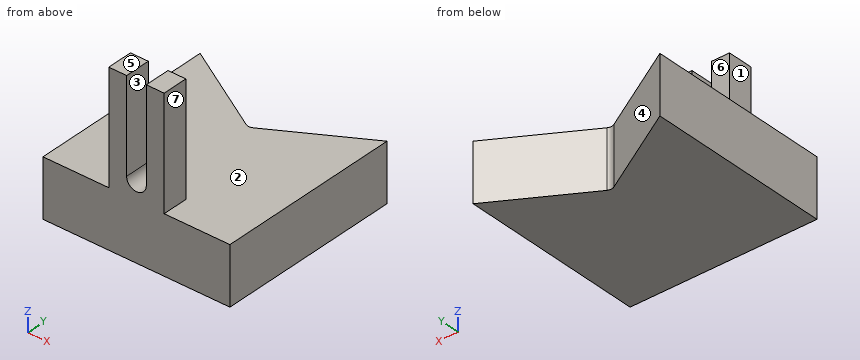
```python
from build123d import *

# Parameters (mm, degrees)
BOSS_EXTRUDE1_DEPTH      = 20.7518
BOSS_EXTRUDE3_DEPTH      = 10
BOSS_EXTRUDE3_DEPTH_BACK = 10
SKETCH6_W                = 40
SKETCH6_H                = 9.27
FILLET1_R                = 2.54
CUT_EXTRUDE11_START      = -47.652475
CUT_EXTRUDE11_DEPTH      = 10


with BuildPart() as part:
    # Sketch1 → Boss-Extrude1 (new body)
    with BuildSketch(Plane.XY):
        Polygon((-33.735, 19.476911331), (0, 0), (33.735, 19.476911331), (33.735, -47.652474646), (-33.735, -47.652474646), align=None)
    extrude(amount=BOSS_EXTRUDE1_DEPTH)

    # Sketch6 → Boss-Extrude3 (add, two sides: drawn at the far end of the back side and taken through both)
    with BuildSketch(Plane(origin=(0, 0, 0), x_dir=(0, 0, -1), z_dir=(1, 0, 0)).offset(-BOSS_EXTRUDE3_DEPTH_BACK)):
        with Locations((-40.7518, -43.017474646)):
            Rectangle(SKETCH6_W, SKETCH6_H)
    extrude(amount=BOSS_EXTRUDE3_DEPTH + BOSS_EXTRUDE3_DEPTH_BACK)

    # Fillet1
    fillet1_edges = [part.edges().sort_by_distance(p)[0] for p in [
        (0, 0, 10.3759),
    ]]
    fillet(fillet1_edges, radius=FILLET1_R)

    # Sketch7 → Cut-Extrude11 (cut)
    with BuildSketch(Plane(origin=(0, 0, 0), x_dir=(1, 0, 0), z_dir=(0, 1, 0)).offset(CUT_EXTRUDE11_START)):
        with BuildLine():
            Line((-3.555, -27.3068), (-3.555, -94.1968))
            ThreePointArc((-3.555, -94.1968), (0, -97.7518), (3.555, -94.1968))
            Line((3.555, -94.1968), (3.555, -27.3068))
            ThreePointArc((3.555, -27.3068), (0, -23.7518), (-3.555, -27.3068))
        make_face()
    extrude(amount=CUT_EXTRUDE11_DEPTH, mode=Mode.SUBTRACT)


solid = part.part
```
Model file for the job. Use its own axes, mm. Face numbers are marked on the shaded views. A direction names the side the tool comes from. Give positions to 0.01 mm unless a question says otherwise; leave off trailing zeros. Order: outer loops, then holes, each group sorted by start corner. A loop starts at its lowest first (then second) coordinate and runs counter-clockwise, first axis right, second up.
1) Wall check: probe 1 along Z at (x, y) = (-21, -14); probe 2 along X at (y, z) = (16.5, 3.5) (3 decimals); probe 3 along Y at (x, z) = (-9.5, 20.5). Give the ranges that are in metal, low to high.
2) Mould opens along X. For the marked faces 1, 2 and 3 say: +X half, -X half, draft (parallel to the pull), parting line (faces both ways), or undercut.
3) Pin check, flat tips, straight feed: pin 1 (3 mm diameter, centred on y = -41, z = 37, fed in from -X); pin 2 (7.5 mm diameter, centred on y = -44, z = 32, fed in from +X); pin 3 (1.5 mm diameter, centred on x = 16, y = -22.5, fed in from +Z). Stop position of each tip, or through.
4) Saw through at B-B, the plane y = 12.5. Write the cut outline in (x, z) (3 decimals).
5) Saw through at A-A, the plane z = 30. Write the cut outline in (x, y) (3 decimals).
6) 3-axis set-ups, long thin cutter, end or side, ignore diameter. For the marked faces 4, 5, 6 and 7: which of +Z, -Z, +X, -X, +Y, -Y reach the whole face in a straight line?
7) Saw through at C-C, the plane x = 0. Write the cut outline in (y, z), then the cut area to 3 significant figures.
8) Saw through at D-D, the plane y = -27.5. Write the cut outline in (x, z) (3 decimals).
Computed:
1. probe 1: z = 0 to 20.75
1. probe 2: x = -33.735 to -28.579, 28.579 to 33.735
1. probe 3: y = -47.65 to 5.48
2. face 1: -X half
2. face 2: draft
2. face 3: undercut
3. pin 1: stops at x = -10
3. pin 2: stops at x = 10
3. pin 3: stops at z = 20.75
4. outline: (-33.735, 0) - (-21.651, 0) - (-21.651, 20.752) - (-33.735, 20.752) - close; (21.651, 0) - (33.735, 0) - (33.735, 20.752) - (21.651, 20.752) - close
5. outline: (-10, -47.652) - (-3.555, -47.652) - (-3.555, -38.382) - (-10, -38.382) - close; (3.555, -47.652) - (10, -47.652) - (10, -38.382) - (3.555, -38.382) - close
6. face 4: +Z, -Z, +Y
6. face 5: +Z, +X, -X, +Y, -Y
6. face 6: +Z, +X, -X, +Y
6. face 7: +Z, +X, +Y, -Y
7. outline: (-47.65, 0) - (0.39, 0) - (0.39, 20.75) - (-38.38, 20.75) - (-38.38, 23.75) - (-47.65, 23.75) - close
7. area: 1,020 mm2
8. outline: (-33.735, 0) - (33.735, 0) - (33.735, 20.752) - (-33.735, 20.752) - close
